Verification items for the finished model (mm, model axes). A direction names the side the tool comes from. Round coordinates to 2 decimals unless told otherwise and drop trailing zeros. Write each loop counter-clockwise with the first axis right and the second up, starting at its lowest first coordinate (ties: lowest second). Pieces come first, ordered by that corner, then holes. Notation, with made-up numbers: (81.5, 59) - (140.5, 59) arc R17 ccw to (140.5, 82) - close; hole circle Ø5 at (-35, -15). An arc over 180 degrees is marked (long way). Write each question's results on one line, items separated by ' | '.
```python
from build123d import *

# Parameters (mm, degrees)
F1_DEPTH = 40
F2_R     = 2.35
F3_DEPTH = 19


with BuildPart() as f1:
    # F0 (on Front) → F1 (new body)
    with BuildSketch(Plane.XZ):
        Polygon((-21, 21), (-21, 0), (-21, -21), (0, -21), (21, -21), (21, 0), (21, 21), (0, 21), align=None)
    extrude(amount=F1_DEPTH)

    # F2 (on face) → F3 (join)
    with BuildSketch(Plane(origin=(0, 0, 0), x_dir=(-1, 0, 0), z_dir=(0, 1, 0))):
        Circle(F2_R)
    extrude(amount=F3_DEPTH)


solid = f1.part
```
(1) Section check B-B (z = 0). Record the cut outline in (x, y).
Answer:
outline: (-21, -40) - (21, -40) - (21, 0) - (2.35, 0) - (2.35, 19) - (-2.35, 19) - (-2.35, 0) - (-21, 0) - close
(2) Section check A-A (x = 0). Record the cut outline in (y, z), plus the area to 3 significant figures.
Answer:
outline: (-40, -21) - (0, -21) - (0, -2.35) - (19, -2.35) - (19, 2.35) - (0, 2.35) - (0, 21) - (-40, 21) - close | area: 1,770 mm2
(3) Go/stop test with flat-tipped pins: pin 1 Ø6 at (x, y) = (-4, 2.5) entering from -Z; pin 2 Ø12 at (x, z) = (2.5, 9) entering from +Y. Record where each tip stops, or that it passes through.
Answer:
pin 1: z = -21 | pin 2: y = 0
(4) Set-up check for faces 1 (the cylindrical face through (0.509, 9.367, -2.294)), 2 (the flat face through (0, -20, 21)): record each of +Z, -Z, +X, -X, +Y, -Y from which the full face is reachable in a straight line by a thin tool's end or side.
Answer:
face 1: +Y | face 2: +Z, +X, -X, +Y, -Y
(5) Thickness scan on L1, parallel to Y at x = 13, z = 3. Record the ranges inside material, lowest first.
Answer:
L1: -40 to 0
(6) Section check D-D (x = -11). Record the cut outline in (y, z), plus the area to 3 significant figures.
Answer:
outline: (-40, -21) - (0, -21) - (0, 21) - (-40, 21) - close | area: 1,680 mm2
(7) Section check C-C (y = 12.5). Record the cut outline in (x, z).
Answer:
outline: circle Ø4.7 at (0, 0)
